The model under review builds one solid part; all positions refer to its coordinate system, in mm. A direction names the side the tool comes from. Coordinates: 2 decimals unless noted, no trailing zeros. Order: outer loops, then holes, each group sorted by start corner. A loop starts at its lowest first (then second) coordinate and runs counter-clockwise, first axis right, second up. Notation, with made-up numbers: (48.5, 21) -> (85.5, 21) arc R14 ccw to (85.5, 48) -> close; hole circle Ø11 at (-6, 35.25). An arc over 180 degrees is marked (long way). Use one line per item in the form item = value.
from build123d import *

# Parameters (mm, degrees)
SKETCH1_R           = 100
BOSS_EXTRUDE1_DEPTH = 40
BOSS_EXTRUDE4_DEPTH = 10


with BuildPart() as part:
    # Sketch1 → Boss-Extrude1 (new body)
    with BuildSketch(Plane.XY):
        Circle(SKETCH1_R)
    extrude(amount=BOSS_EXTRUDE1_DEPTH)

    # Sketch3 → Boss-Extrude4 (add)
    with BuildSketch(Plane.XY):
        Polygon((-0.602668663, 0.79799153), (-36.821347212, -26.555510029), (-38.629353201, -24.161535438), (-60.970804607, -46.04709685), (-33.808003897, -30.545467681), (-35.616009886, -28.15149309), (0.602668663, -0.79799153), align=None)
        with BuildLine():
            Line((-1.602668663, 99.861033349), (-1.602668663, 82.422716301))
            ThreePointArc((-1.602668663, 82.422716301), (-0.602668663, 81.422716301), (0.397331337, 82.422716301))
            Line((0.397331337, 82.422716301), (0.397331337, 99.861033349))
            Line((0.397331337, 99.861033349), (-1.602668663, 99.861033349))
        make_face()
        with BuildLine():
            Line((48.542564899, 87.28352606), (39.823406374, 72.181500497))
            ThreePointArc((39.823406374, 72.181500497), (40.189431778, 70.815475093), (41.555457182, 71.181500497))
            Line((41.555457182, 71.181500497), (50.274615706, 86.28352606))
            Line((50.274615706, 86.28352606), (48.542564899, 87.28352606))
        make_face()
        with BuildLine():
            Line((85.680857397, 51.318468451), (70.578831834, 42.599309926))
            ThreePointArc((70.578831834, 42.599309926), (70.21280643, 41.233284522), (71.578831834, 40.867259119))
            Line((71.578831834, 40.867259119), (86.680857397, 49.586417643))
            Line((86.680857397, 49.586417643), (85.680857397, 51.318468451))
        make_face()
        with BuildLine():
            Line((99.861033349, 1.602668663), (82.422716301, 1.602668663))
            ThreePointArc((82.422716301, 1.602668663), (81.422716301, 0.602668663), (82.422716301, -0.397331337))
            Line((82.422716301, -0.397331337), (99.861033349, -0.397331337))
            Line((99.861033349, -0.397331337), (99.861033349, 1.602668663))
        make_face()
        with BuildLine():
            Line((87.28352606, -48.542564899), (72.181500497, -39.823406374))
            ThreePointArc((72.181500497, -39.823406374), (70.815475093, -40.189431778), (71.181500497, -41.555457182))
            Line((71.181500497, -41.555457182), (86.28352606, -50.274615706))
            Line((86.28352606, -50.274615706), (87.28352606, -48.542564899))
        make_face()
        with BuildLine():
            Line((51.318468451, -85.680857397), (42.599309926, -70.578831834))
            ThreePointArc((42.599309926, -70.578831834), (41.233284522, -70.21280643), (40.867259119, -71.578831834))
            Line((40.867259119, -71.578831834), (49.586417643, -86.680857397))
            Line((49.586417643, -86.680857397), (51.318468451, -85.680857397))
        make_face()
        with BuildLine():
            Line((1.602668663, -99.861033349), (1.602668663, -82.422716301))
            ThreePointArc((1.602668663, -82.422716301), (0.602668663, -81.422716301), (-0.397331337, -82.422716301))
            Line((-0.397331337, -82.422716301), (-0.397331337, -99.861033349))
            Line((-0.397331337, -99.861033349), (1.602668663, -99.861033349))
        make_face()
        with BuildLine():
            Line((-48.542564899, -87.28352606), (-39.823406374, -72.181500497))
            ThreePointArc((-39.823406374, -72.181500497), (-40.189431778, -70.815475093), (-41.555457182, -71.181500497))
            Line((-41.555457182, -71.181500497), (-50.274615706, -86.28352606))
            Line((-50.274615706, -86.28352606), (-48.542564899, -87.28352606))
        make_face()
        with BuildLine():
            Line((-85.680857397, -51.318468451), (-70.578831834, -42.599309926))
            ThreePointArc((-70.578831834, -42.599309926), (-70.21280643, -41.233284522), (-71.578831834, -40.867259119))
            Line((-71.578831834, -40.867259119), (-86.680857397, -49.586417643))
            Line((-86.680857397, -49.586417643), (-85.680857397, -51.318468451))
        make_face()
        with BuildLine():
            Line((-99.861033349, -1.602668663), (-82.422716301, -1.602668663))
            ThreePointArc((-82.422716301, -1.602668663), (-81.422716301, -0.602668663), (-82.422716301, 0.397331337))
            Line((-82.422716301, 0.397331337), (-99.861033349, 0.397331337))
            Line((-99.861033349, 0.397331337), (-99.861033349, -1.602668663))
        make_face()
        with BuildLine():
            Line((-87.28352606, 48.542564899), (-72.181500497, 39.823406374))
            ThreePointArc((-72.181500497, 39.823406374), (-70.815475093, 40.189431778), (-71.181500497, 41.555457182))
            Line((-71.181500497, 41.555457182), (-86.28352606, 50.274615706))
            Line((-86.28352606, 50.274615706), (-87.28352606, 48.542564899))
        make_face()
        with BuildLine():
            Line((-51.318468451, 85.680857397), (-42.599309926, 70.578831834))
            ThreePointArc((-42.599309926, 70.578831834), (-41.233284522, 70.21280643), (-40.867259119, 71.578831834))
            Line((-40.867259119, 71.578831834), (-49.586417643, 86.680857397))
            Line((-49.586417643, 86.680857397), (-51.318468451, 85.680857397))
        make_face()
    extrude(amount=-BOSS_EXTRUDE4_DEPTH)


solid = part.part
Item 1: We need section D-D (y = 10.5). Write out the cut boundary in (x, z).
Results found:
outline = (-99.45, 0) -> (99.45, 0) -> (99.45, 40) -> (-99.45, 40) -> close
Item 2: Draft analysis for pull direction Y (two halves, no side actions). For faces 5 (the face through (-0.397, -91, -5)), 6 (the face through (79.838, -44.244, -4.93)), 7 (the face through (44.244, 79.838, -4.93)), state which applies: released by +Y, released by -Y, zero draft, split by the parting line, or undercut.
Results found:
face_5 = zero draft
face_6 = undercut
face_7 = released by +Y
Item 3: We need section A-A (x = -27). Write out the cut boundary in (y, z).
Results found:
outline = (-96.29, 0) -> (-21.64, 0) -> (-21.64, -10) -> (-19.14, -10) -> (-19.14, 0) -> (96.29, 0) -> (96.29, 40) -> (-96.29, 40) -> close
Item 4: To check wall thickness, follow L1, parallel to Y at x = -48, z = -5; L2, parallel to Z at x = -40.5, y = -49; L3, parallel to Y at x = 46, z = -7. State the ranges of each line that lie inside material, in increasing order. Write a range as from..to.
Results found:
L1 = -86.34..-82.34, -38.64..-33.34, 79.93..83.93
L2 = 0..40
L3 = -80.47..-76.47, 78.88..82.88
Item 5: Clearance check with flat-ended pins moving along their axes: pin 1 (3 mm diameter, centred on x = 92.5, z = -3, fed in from -Y); pin 2 (8 mm diameter, centred on x = 63.5, y = 43.5, fed in from -Z); pin 3 (12 mm diameter, centred on y = -58, z = -4.5, fed in from +X). State where each tip first meets the part, or that it passes through.
Results found:
pin_1 = -0.4
pin_2 = 0
pin_3 = 84.15
Item 6: Tool access review of faces 1 (the face through (47, -78.2, -4.9)), 2 (the face through (-91, 0.397, -5)), 3 (the face through (78.627, -45.854, -4.93)), 4 (the face through (-78.627, 45.854, -4.93)): name each direction out of +Z, -Z, +X, -X, +Y, -Y from which nothing blocks a thin tool from reaching the whole face with its end or side.
Results found:
face_1 = -Z, +X
face_2 = -Z, -X
face_3 = -Z, -Y
face_4 = -Z, +Y
Item 7: We need section B-B (z = 32). Write out the cut boundary in (x, y).
Results found:
outline = circle Ø200 at (0, 0)
Item 8: We need section C-C (y = 31.5). Write out the cut boundary in (x, z), plus the area to 3 significant figures.
Results found:
outline = (-94.91, 0) -> (94.91, 0) -> (94.91, 40) -> (-94.91, 40) -> close
area = 7,590 mm²
